Build history of the part. All positions in model axes, mm. A direction names the side the tool comes from. Round coordinates to 2 decimals unless told otherwise and drop trailing zeros. Write each loop counter-clockwise with the first axis right and the second up, starting at its lowest first coordinate (ties: lowest second). Pieces come first, ordered by that corner, then holes. Notation, with made-up numbers: (28, 69) - (51, 69) arc R8 cw to (51, 79) - close; hole circle Ø3 at (35.5, 45.5). An arc over 180 degrees is marked (long way). One line per question, with ' | ' between items.
Autodesk Inventor part; units mm, degrees
ref_plane "YZ Plane" through (0, 0, 0) normal (1, 0, 0) x (0, 1, 0)
ref_plane "XZ Plane" through (0, 0, 0) normal (0, 1, 0) x (-1, 0, 0)
ref_plane "XY Plane" through (0, 0, 0) normal (0, 0, 1) x (1, 0, 0)
sketch "Sketch1" plane through (0, 0, 0) normal (0, 0, 1) x (1, 0, 0)
  circle A0 centre (0, 0) radius 6.75
  dimension "d0" = 13.5
extrude "Extrusion1" add sketch "Sketch1" along normal blind 15
sketch "Sketch2" plane through (0, 0, 15) normal (0, 0, 1) x (1, 0, 0)
  circle A0 centre (0, 0) radius 11.15
  circle A1 centre (0, 0) radius 12.75
  dimension "d3" = 22.3
  dimension "d19" = 25.5
extrude "Extrusion3" add sketch "Sketch2" along normal blind 5 contours A0
sketch "Sketch3" plane through (0, 0, 15) normal (0, 0, -1) x (-1, 0, 0)
  circle A0 centre (0, 0) radius 10.15
  circle A1 centre (0, 0) radius 11.15
  dimension "d8" = 20.3
  dimension "d9" = 22.3
extrude "Extrusion4" add sketch "Sketch3" along normal blind 5
sketch "Sketch4" plane through (0, 0, 20) normal (0, 0, 1) x (1, 0, 0)
  circle A0 centre (0, 0) radius 14.25
  dimension "d12" = 28.5
extrude "Extrusion5" [suppressed]
fillet "Fillet1" [suppressed]
fillet "Fillet2" radius 2 1 edges at (-6.75, 0, 0)
fillet "Fillet3" radius 2 1 edges at (11.15, 0, 10)
fillet "Fillet4" [suppressed]
sketch "Sketch7" plane through (0, 0, 20) normal (0, 0, 1) x (1, 0, 0)
  circle A0 centre (0, 0) radius 15
  dimension "d20" = 30
extrude "Extrusion6" add sketch "Sketch7" along normal blind 2
sketch "Sketch8" plane through (0, 0, 22) normal (0, 0, 1) x (1, 0, 0)
  circle A0 centre (0, 0) radius 11.25
  circle A1 centre (0, 0) radius 15
  dimension "d23" = 22.5
  dimension "d24" = 30
extrude "Extrusion7" add sketch "Sketch8" along normal blind 10
properties part number "Elbow_Parallel_Rod_V1"
Q1. Which spindle directions (+Z, -Z, +X, -X, +Y, -Y) get a long thin tool onto all of the face, cutting with end or side? Do faces 4 (the cylindrical face through (5.19, 9.98, 26.93)), 5 (the cylindrical face through (8.05, 6.18, 12.54)), 6 (the flat face through (2.2, 11.2, 32)). Say none if no direction does.
Found:
face 4: +Z | face 5: -Z | face 6: +Z, +X, -X, +Y, -Y
Q2. Saw through at D-D, the plane z = 18. List the corners of the cut face in (x, y), then the cut area to 3 significant figures.
Found:
outline: circle Ø22.3 at (0, 0) | area: 391 mm^2
Q3. Saw through at A-A, the plane x = 0. List the corners of the cut face in (y, z).
Found:
outline: (-15, 20) - (-11.15, 20) - (-11.15, 11.73) arc R2 ccw to (-10.15, 10) - (-10.15, 15) - (-6.75, 15) - (-6.75, 2) arc R2 ccw to (-4.75, 0) - (4.75, 0) arc R2 ccw to (6.75, 2) - (6.75, 15) - (10.15, 15) - (10.15, 10) arc R2 ccw to (11.15, 11.73) - (11.15, 20) - (15, 20) - (15, 32) - (11.25, 32) - (11.25, 22) - (-11.25, 22) - (-11.25, 32) - (-15, 32) - close
Q4. Saw through at C-C, the plane z = 29.5. List the corners of the cut face in (x, y).
Found:
outline: circle Ø30 at (0, 0); hole circle Ø22.5 at (0, 0)
Q5. Drill centre lines: L1, parallel to Y at x = 0, z = 29.5; L2, parallel to Y at x = 0, z = 11.2; L3, parallel to Z at x = -0.25, y = 4.75. Where is each one in solid material? Low to high. Write a range as from..to.
Found:
L1: -15..-11.25, 11.25..15 | L2: -11.08..-10.15, -6.75..6.75, 10.15..11.08 | L3: 0..22
Q6. Drop flat-ended pins along their axis: pin 1 (10 mm diameter, centred on x = 10, z = 3.5, fed in from +Y); pin 2 (5 mm diameter, centred on y = 1, z = 6, fed in from +X); pin 3 (6 mm diameter, centred on x = -9, z = 16.5, fed in from -Y). Give the stop position or say it passes through.
Found:
pin 1: y = 4.53 | pin 2: x = 6.75 | pin 3: y = -9.4
Q7. Pull direction Y, two halves, no side cores. Call faces 1 (the flat face through (0, 0, 0)), 2 (the cylindrical face through (-14.985, -0.66, 25.916)), 3 (the flat face through (2, -7, 15)): +Y half, -Y half, draft (parallel to the pull), parting line (faces both ways), or undercut.
Found:
face 1: draft | face 2: parting line | face 3: undercut
